from build123d import *

# Parameters (mm, degrees)
SKETCH1_W           = 50
SKETCH1_H           = 50
BOSS_EXTRUDE1_DEPTH = 1.6
SKETCH2_W           = 46.8
SKETCH2_H           = 46.8
SKETCH2_W_2         = 43.6
SKETCH2_H_2         = 43.6
BOSS_EXTRUDE2_DEPTH = 4
FILLET1_R           = 5


with BuildPart() as part:
    # Sketch1 → Boss-Extrude1 (new body)
    with BuildSketch(Plane(origin=(0, 0, 0), x_dir=(1, 0, 0), z_dir=(0, 1, 0))):
        Rectangle(SKETCH1_W, SKETCH1_H)
    extrude(amount=BOSS_EXTRUDE1_DEPTH)

    # Sketch2 → Boss-Extrude2 (add)
    with BuildSketch(Plane(origin=(0, 1.6, 0), x_dir=(1, 0, 0), z_dir=(0, 1, 0))):
        Rectangle(SKETCH2_W, SKETCH2_H)
        Rectangle(SKETCH2_W_2, SKETCH2_H_2, mode=Mode.SUBTRACT)
    extrude(amount=BOSS_EXTRUDE2_DEPTH)

    # Fillet1
    fillet1_edges = [part.edges().sort_by_distance(p)[0] for p in [
        (-23.4, 3.6, 23.4),
        (23.4, 3.6, 23.4),
        (23.4, 3.6, -23.4),
        (-23.4, 3.6, -23.4),
        (21.8, 3.6, 21.8),
        (21.8, 3.6, -21.8),
        (-21.8, 3.6, -21.8),
        (-21.8, 3.6, 21.8),
        (25, 0.8, 25),
        (-25, 0.8, 25),
        (-25, 0.8, -25),
        (25, 0.8, -25),
    ]]
    fillet(fillet1_edges, radius=FILLET1_R)


solid = part.part
For this review, take the finished solid that the model builds, in its own axes (mm). A direction names the side the tool comes from. Coordinates: 2 decimals unless noted, no trailing zeros. Order: outer loops, then holes, each group sorted by start corner. A loop starts at its lowest first (then second) coordinate and runs counter-clockwise, first axis right, second up. Notation, with made-up numbers: (69, -0.5) -> (94, -0.5) arc R18 cw to (94, 14.5) -> close; hole circle Ø3 at (-9, 46.25). An arc over 180 degrees is marked (long way). Return JSON: item names as keys, results as strings.
1. We need section C-C on z = 0. Write out the cut boundary in (x, y).
Answer block:
{"outline": "(-25, 0) -> (25, 0) -> (25, 1.6) -> (23.4, 1.6) -> (23.4, 5.6) -> (21.8, 5.6) -> (21.8, 1.6) -> (-21.8, 1.6) -> (-21.8, 5.6) -> (-23.4, 5.6) -> (-23.4, 1.6) -> (-25, 1.6) -> close"}
2. We need section A-A on y = 2.75. Write out the cut boundary in (x, z), and give its area (3 significant figures).
Answer block:
{"outline": "(-23.4, -18.4) arc R5 ccw to (-18.4, -23.4) -> (18.4, -23.4) arc R5 ccw to (23.4, -18.4) -> (23.4, 18.4) arc R5 ccw to (18.4, 23.4) -> (-18.4, 23.4) arc R5 ccw to (-23.4, 18.4) -> close; hole (-21.8, -16.8) arc R5 ccw to (-16.8, -21.8) -> (16.8, -21.8) arc R5 ccw to (21.8, -16.8) -> (21.8, 16.8) arc R5 ccw to (16.8, 21.8) -> (-16.8, 21.8) arc R5 ccw to (-21.8, 16.8) -> close", "area": "289 mm²"}
3. Machinability: for faces 5 (the flat face through (-23.4, 4, 0)), 6 (the flat face through (0, 4, -23.4)), 7 (the flat face through (-2, 1.6, 24)), which of the approach directions +Z, -Z, +X, -X, +Y, -Y give a long, thin tool a straight path to every point of the face, cutting with its end or side? Answer none if there is none.
Answer block:
{"face 5": "+Z, -Z, -X, +Y", "face 6": "-Z, +X, -X, +Y", "face 7": "+Y"}
4. We need section B-B on x = -16. Write out the cut boundary in (y, z), and give its area (3 significant figures).
Answer block:
{"outline": "(0, -25) -> (1.6, -25) -> (1.6, -23.4) -> (5.6, -23.4) -> (5.6, -21.8) -> (1.6, -21.8) -> (1.6, 21.8) -> (5.6, 21.8) -> (5.6, 23.4) -> (1.6, 23.4) -> (1.6, 25) -> (0, 25) -> close", "area": "92.8 mm²"}
5. For line 1 (X direction, y = 2.65, z = -11.5); line 2 (Y direction, x = -17.5, z = 13.5), list the stretches that pass through material, from the lowest coordinate up. Write a range as from..to.
Answer block:
{"line 1": "-23.4..-21.8, 21.8..23.4", "line 2": "0..1.6"}
6. The part is to be moulded in two halves that separate along Z. For faces 1 (the cylindrical face through (20.3, 3.63, 20.37)), 2 (the flat face through (-2, 5.6, 22)), 3 (the cylindrical face through (-24, 1, -23)), 4 (the flat face through (0, 1.6, 0)), say which applies: +Z half, -Z half, draft (parallel to the pull), parting line (faces both ways), or undercut.
Answer block:
{"face 1": "undercut", "face 2": "draft", "face 3": "-Z half", "face 4": "undercut"}
7. For pin 1 Ø1.2 at (x, y) = (-8, 4) entering from -Z; pin 2 Ø2 at (x, z) = (-17.5, -19.5) entering from +Y; pin 3 Ø2 at (y, z) = (3.5, -6) entering from +X, all flat-tipped, find the tip position at first contact; note any pin that passes through.
Answer block:
{"pin 1": "z = -23.4", "pin 2": "y = 1.6", "pin 3": "x = 23.4"}
